The drawing under review shows one solid part. Ordinate dimensions are in mm from its lowest x, y, z. Coordinates: 2 decimals unless noted, no trailing zeros. Write each loop counter-clockwise with the first axis right and the second up, starting at its lowest first coordinate (ties: lowest second). Pieces come first, ordered by that corner, then holes.
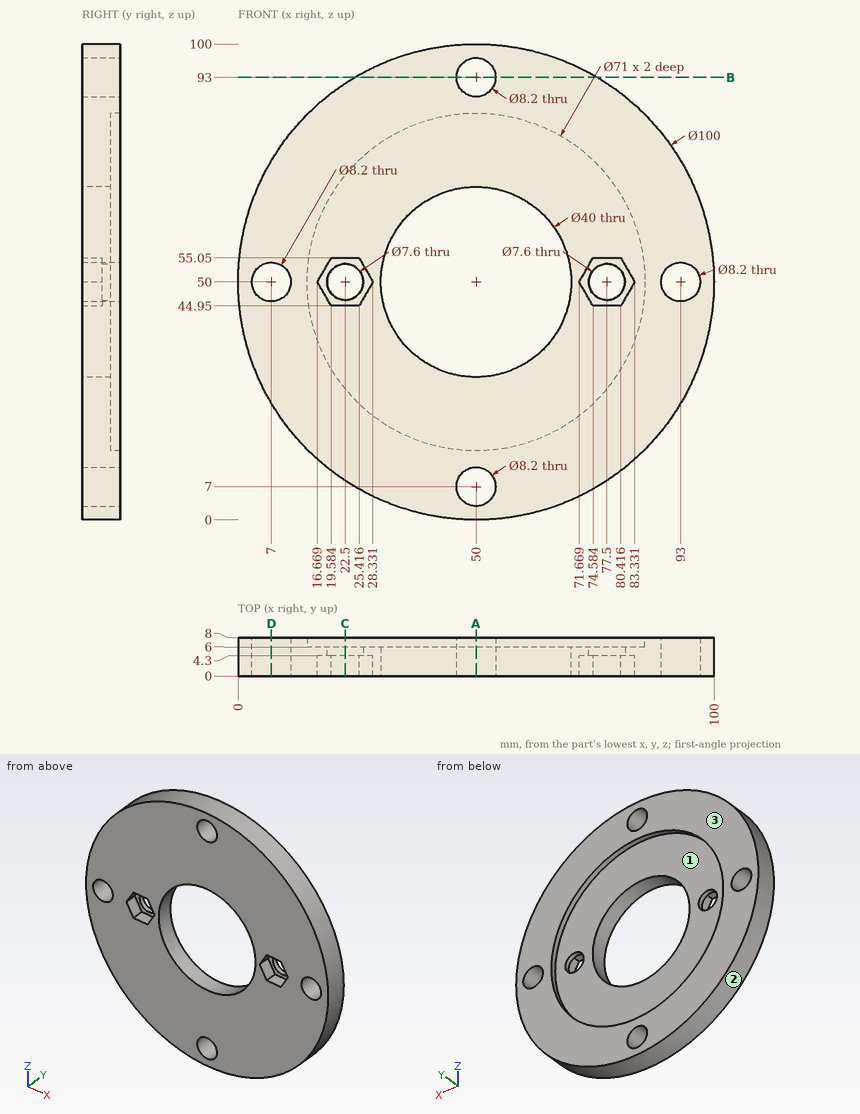
Q1. Draft analysis for pull direction Z (two halves, no side actions). For the marked faces 1, 2 and 3, state which applies: +Z half, -Z half, draft (parallel to the pull), parting line (faces both ways), or undercut.
Ans:
face 1: undercut
face 2: parting line
face 3: draft
Q2. Add section A-A (x = 50). State the section outline as (y, z) points.
Ans:
outline: (0, 0) - (8, 0) - (8, 2.9) - (0, 2.9) - close; (0, 11.1) - (8, 11.1) - (8, 14.5) - (6, 14.5) - (6, 30) - (0, 30) - close; (0, 70) - (6, 70) - (6, 85.5) - (8, 85.5) - (8, 88.9) - (0, 88.9) - close; (0, 97.1) - (8, 97.1) - (8, 100) - (0, 100) - close
Q3. Add section D-D (x = 7). State the section outline as (y, z) points (1 decimal), then the cut area to 3 significant figures.
Ans:
outline: (0, 24.5) - (8, 24.5) - (8, 45.9) - (0, 45.9) - close; (0, 54.1) - (8, 54.1) - (8, 75.5) - (0, 75.5) - close
area: 343 mm2
Q4. Add section B-B (z = 93). State the section outline as (x, y) points (1 decimal), then the cut area to 3 significant figures.
Ans:
outline: (24.5, 0) - (45.9, 0) - (45.9, 8) - (24.5, 8) - close; (54.1, 0) - (75.5, 0) - (75.5, 8) - (54.1, 8) - close
area: 343 mm2
Q5. Add section C-C (x = 22.5). State the section outline as (y, z) points, then the cut area to 3 significant figures.
Ans:
outline: (0, 8.24) - (8, 8.24) - (8, 27.55) - (6, 27.55) - (6, 46.2) - (4.3, 46.2) - (4.3, 44.95) - (0, 44.95) - close; (0, 55.05) - (4.3, 55.05) - (4.3, 53.8) - (6, 53.8) - (6, 72.45) - (8, 72.45) - (8, 91.76) - (0, 91.76) - close
area: 522 mm2
Q6. For probe 1 along X at (y, z) = (6.25, 50); probe 2 along X at (y, z) = (1.5, 54.5), list the stretches that pass through material, from the lowest coordinate up.
Ans:
probe 1: x = 0 to 2.9, 11.1 to 14.5, 85.5 to 88.9, 97.1 to 100
probe 2: x = 0.2 to 19.27, 25.73 to 30.51, 69.49 to 74.27, 80.73 to 99.8
Q7. Clearance check with flat-ended pins moving along their axes: pin 1 Ø3 at (y, z) = (7, 12) entering from -X; pin 2 Ø1 at (y, z) = (2, 86) entering from -X; pin 3 Ø3 at (y, z) = (4, 74.5) entering from +X (1 decimal). State where each tip first meets the part, or that it passes through.
Ans:
pin 1: stops at x = 15.83
pin 2: stops at x = 14.79
pin 3: stops at x = 94.4
